```python
from build123d import *

# Parameters (mm, degrees)
SKETCH2_R          = 1.5
CUT_EXTRUDE1_DEPTH = 60.56828015


with BuildPart() as part:
    # Sketch1 → Revolve1 (revolve)
    with BuildSketch(Plane.XY, mode=Mode.PRIVATE) as revolve1_sk:
        Polygon((0, -12.7), (30.5054, 6.35), (31.75, 6.35), (31.75, 0), (38.1, 0), (38.1, -19.05), (0, -19.05), align=None)
    revolve(revolve1_sk.sketch.rotate(Axis((0, -19.05, 0), (0, 1, 0)), 90), axis=Axis((0, -19.05, 0), (0, 1, 0)))

    # Sketch2 → Cut-Extrude1 (cut, through all)
    with BuildSketch(Plane.XZ.offset(19.05)):
        with Locations(Location((0, 0, 0), (0, 0, 270))):
            Circle(SKETCH2_R)
    extrude(amount=-CUT_EXTRUDE1_DEPTH, mode=Mode.SUBTRACT)


solid = part.part
```
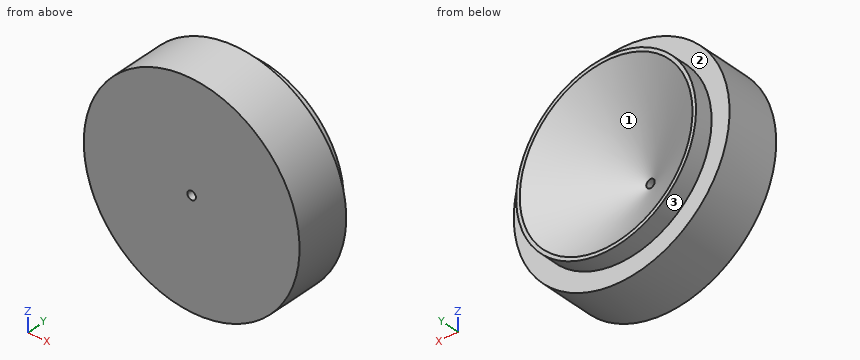
Part model, mm, in its own coordinate system. Face numbers are marked on the shaded views. Coordinates: 2 decimals unless noted, no trailing zeros. Write each loop counter-clockwise with the first axis right and the second up, starting at its lowest first coordinate (ties: lowest second). Pieces come first, ordered by that corner, then holes.
Item 1: Slice it at A-A (z = 0). Write the cut outline in (x, y), and give its area (3 significant figures).
Item 2: Pin check, flat tips, straight feed: pin 1 (6 mm diameter, centred on y = 3.5, z = -3, fed in from -X); pin 2 (2 mm diameter, centred on y = -11, z = 19, fed in from -X); pin 3 (1 mm diameter, centred on x = 23.5, z = 4.5, fed in from +Y); pin 4 (2.5 mm diameter, centred on x = 0, z = 0, fed in from +Y). Stop position of each tip, or through.
Item 3: Slice it at B-B (x = 0). Write the cut outline in (y, z).
Item 4: Slice it at D-D (y = 4.75). Write the cut outline in (x, z), and give its area (3 significant figures).
Item 5: Slice it at C-C (y = -1.75). Write the cut outline in (x, z), and give its area (3 significant figures).
Item 6: Mould opens along Z. For the marked faces 1, 2 and 3 say: released by +Z, released by -Z, zero draft, split by the parting line, or undercut.
Item 7: Probe line 1 (X direction, y = -16.75, z = 0); line 2 (Z direction, x = 12, y = 2); line 3 (Y direction, x = -33, z = 14.5). List the from-to ranges inside material, lowest first.
Results found:
1. outline: (-38.1, -19.05) - (-1.5, -19.05) - (-1.5, -11.76) - (-30.51, 6.35) - (-31.75, 6.35) - (-31.75, 0) - (-38.1, 0) - close; (1.5, -19.05) - (38.1, -19.05) - (38.1, 0) - (31.75, 0) - (31.75, 6.35) - (30.51, 6.35) - (1.5, -11.76) - close
1. area: 1,250 mm2
2. pin 1: stops at x = -31.75
2. pin 2: stops at x = -33.58
2. pin 3: stops at y = 2.55
2. pin 4: passes through
3. outline: (-19.05, -38.1) - (0, -38.1) - (0, -31.75) - (6.35, -31.75) - (6.35, -30.51) - (-11.76, -1.5) - (-19.05, -1.5) - close; (-19.05, 1.5) - (-11.76, 1.5) - (6.35, 30.51) - (6.35, 31.75) - (0, 31.75) - (0, 38.1) - (-19.05, 38.1) - close
4. outline: circle Ø63.5 at (0, 0); hole circle Ø55.89 at (0, 0)
4. area: 714 mm2
5. outline: circle Ø76.2 at (0, 0); hole circle Ø35.07 at (0, 0)
5. area: 3,590 mm2
6. face 1: undercut
6. face 2: zero draft
6. face 3: split by the parting line
7. line 1: x = -38.1 to -1.5, 1.5 to 38.1
7. line 2: z = -29.39 to -20.25, 20.25 to 29.39
7. line 3: y = -19.05 to 0
